The drawing under review shows one solid part. Ordinate dimensions are in mm from its lowest x, y, z. A direction names the side the tool comes from. Coordinates: 2 decimals unless noted, no trailing zeros. Write each loop counter-clockwise with the first axis right and the second up, starting at its lowest first coordinate (ties: lowest second). Pieces come first, ordered by that corner, then holes. Notation, with made-up numbers: (7, 4.5) -> (42, 4.5) arc R9 cw to (42, 12.5) -> close; hole circle Ø11 at (78, 75). An arc over 180 degrees is marked (long way). One line per item, written item: value. Start each with the question number.
1) Add section A-A (z = 8). State the section outline as (x, y) points.
2) For probe 1 along Z at (x, y) = (46.5, 2); probe 2 along X at (y, z) = (24.5, 14.5), list the stretches that pass through material, from the lowest coordinate up. Write a range as from..to.
3) Add section C-C (y = 19.5). State the section outline as (x, z) points, and give its area (3 significant figures).
4) Add section B-B (x = 43). State the section outline as (y, z) points.
5) Mouldability with a two-part tool opening along X and no side actions: class the marked faces 1, 2, 3 and 4 as released by +X, released by -X, zero draft, split by the parting line, or undercut.
6) Machinability: for the marked faces 5 and 6, which of the approach directions +Z, -Z, +X, -X, +Y, -Y give a long, thin tool a straight path to every point of the face, cutting with its end or side? Answer none if there is none.
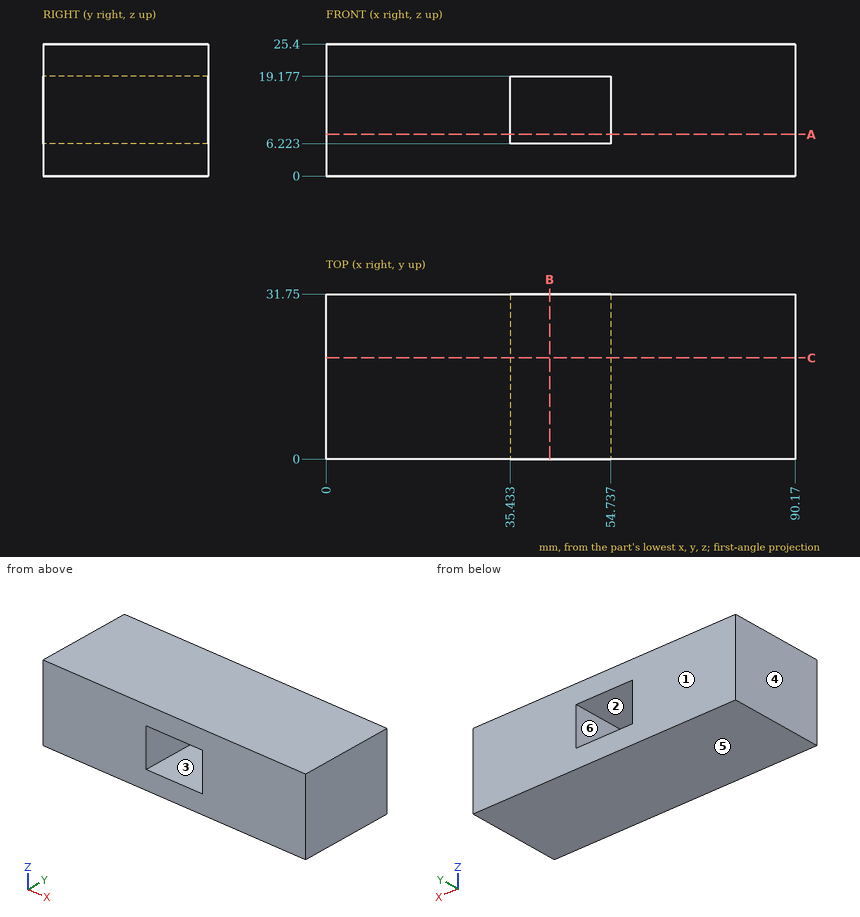
Numbers:
1. outline: (0, 0) -> (35.43, 0) -> (35.43, 31.75) -> (0, 31.75) -> close; (54.74, 0) -> (90.17, 0) -> (90.17, 31.75) -> (54.74, 31.75) -> close
2. probe 1: 0..6.22, 19.18..25.4
2. probe 2: 0..35.43, 54.74..90.17
3. outline: (0, 0) -> (90.17, 0) -> (90.17, 25.4) -> (0, 25.4) -> close; hole (35.43, 6.22) -> (54.74, 6.22) -> (54.74, 19.18) -> (35.43, 19.18) -> close
3. area: 2,040 mm²
4. outline: (0, 0) -> (31.75, 0) -> (31.75, 6.22) -> (0, 6.22) -> close; (0, 19.18) -> (31.75, 19.18) -> (31.75, 25.4) -> (0, 25.4) -> close
5. face 1: zero draft
5. face 2: undercut
5. face 3: undercut
5. face 4: released by -X
6. face 5: -Z, +X, -X, +Y, -Y
6. face 6: +Y, -Y
